from build123d import *

# Parameters (mm, degrees)
SKETCH1_W           = 880
SKETCH1_H           = 580
BOSS_EXTRUDE1_DEPTH = 35
SKETCH2_R           = 50
CUT_EXTRUDE1_DEPTH  = 10
SKETCH3_R           = 30
CUT_EXTRUDE2_DEPTH  = 20
SKETCH4_R           = 15
CUT_EXTRUDE3_DEPTH  = 522
CHAMFER1_SIZE       = 2
SKETCH5_R           = 20
CUT_EXTRUDE4_DEPTH  = 450


with BuildPart() as part:
    # Sketch1 → Boss-Extrude1 (new body)
    with BuildSketch(Plane(origin=(0, 0, 0), x_dir=(1, 0, 0), z_dir=(0, 1, 0))):
        Rectangle(SKETCH1_W, SKETCH1_H)
    extrude(amount=BOSS_EXTRUDE1_DEPTH)

    # Sketch2 → Cut-Extrude1 (cut)
    with BuildSketch(Plane(origin=(0, 35, 0), x_dir=(1, 0, 0), z_dir=(0, 1, 0))):
        with Locations(Location((0, 0, 0), (0, 0, 270))):
            Circle(SKETCH2_R)
    extrude(amount=-CUT_EXTRUDE1_DEPTH, mode=Mode.SUBTRACT)

    # Sketch3 → Cut-Extrude2 (cut)
    with BuildSketch(Plane(origin=(0, 25, 0), x_dir=(1, 0, 0), z_dir=(0, 1, 0))):
        with Locations(Location((0, 0, 0), (0, 0, 270))):
            Circle(SKETCH3_R)
    extrude(amount=-CUT_EXTRUDE2_DEPTH, mode=Mode.SUBTRACT)

    # Sketch4 → Cut-Extrude3 (cut)
    with BuildSketch(Plane(origin=(0, 5, 0), x_dir=(1, 0, 0), z_dir=(0, 1, 0))):
        with Locations(Location((0, 0, 0), (0, 0, 270))):
            Circle(SKETCH4_R)
    extrude(amount=-CUT_EXTRUDE3_DEPTH, mode=Mode.SUBTRACT)

    # Chamfer1
    chamfer1_edges = [part.edges().sort_by_distance(p)[0] for p in [
        (0, 5, -30),
    ]]
    chamfer(chamfer1_edges, length=CHAMFER1_SIZE)

    # Sketch5 → Cut-Extrude4 (cut)
    with BuildSketch(Plane(origin=(0, 35, 0), x_dir=(1, 0, 0), z_dir=(0, 1, 0))):
        with Locations(Location((-340, 200, 0), (0, 0, 270))):
            Circle(SKETCH5_R)
        with Locations(Location((340, 200, 0), (0, 0, 270))):
            Circle(SKETCH5_R)
        with Locations(Location((340, -200, 0), (0, 0, 270))):
            Circle(SKETCH5_R)
        with Locations(Location((-340, -200, 0), (0, 0, 270))):
            Circle(SKETCH5_R)
    extrude(amount=-CUT_EXTRUDE4_DEPTH, mode=Mode.SUBTRACT)


solid = part.part
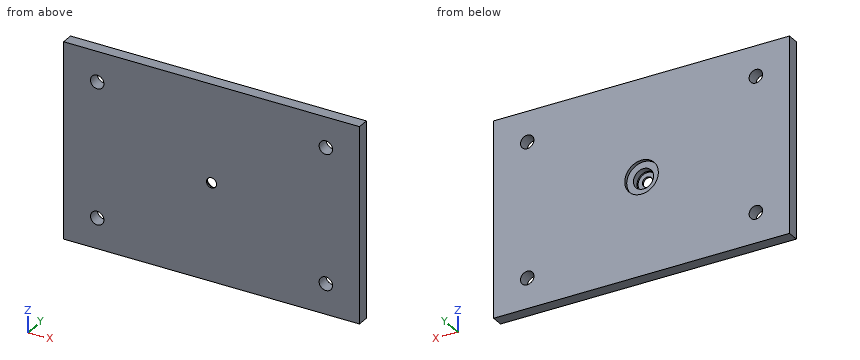
Geometry check sheet. Reference: the model listing, model coordinates, mm. Round coordinates to 2 decimals unless told otherwise and drop trailing zeros. Loops run counter-clockwise (first coordinate to the right, second up) from the corner with the lowest first, then second, coordinate; pieces in that order, holes last.
Item 1: Cross-section at C-C on x = 340. Record the boundary of the cut face in (y, z).
Item 2: Cross-section at A-A on z = 0. Record the boundary of the cut face in (x, y).
Item 3: Thickness scan on line 1 (X direction, y = 16, z = -200); line 2 (X direction, y = 32, z = 0); line 3 (Z direction, x = 335.5, y = 32). Record the ranges inside material, lowest first.
Item 4: Cross-section at D-D on x = 0. Record the boundary of the cut face in (y, z), then the cut area to 3 significant figures.
Item 5: Cross-section at B-B on z = 200. Record the boundary of the cut face in (x, y), then the cut area to 3 significant figures.
Item 6: Gauge pin test, flat end, axial feed: pin 1 (17 mm diameter, centred on x = 3, z = -3.5, fed in from +Y). Record the tip position at first contact, or that the pin passes through.
Answer sheet:
1. outline: (0, -290) - (35, -290) - (35, -220) - (0, -220) - close; (0, -180) - (35, -180) - (35, 180) - (0, 180) - close; (0, 220) - (35, 220) - (35, 290) - (0, 290) - close
2. outline: (-440, 0) - (-15, 0) - (-15, 5) - (-28, 5) - (-30, 7) - (-30, 25) - (-50, 25) - (-50, 35) - (-440, 35) - close; (15, 0) - (440, 0) - (440, 35) - (50, 35) - (50, 25) - (30, 25) - (30, 7) - (28, 5) - (15, 5) - close
3. line 1: x = -440 to -360, -320 to 320, 360 to 440
3. line 2: x = -440 to -50, 50 to 440
3. line 3: z = -290 to -219.49, -180.51 to 180.51, 219.49 to 290
4. outline: (0, -290) - (35, -290) - (35, -50) - (25, -50) - (25, -30) - (7, -30) - (5, -28) - (5, -15) - (0, -15) - close; (0, 15) - (5, 15) - (5, 28) - (7, 30) - (25, 30) - (25, 50) - (35, 50) - (35, 290) - (0, 290) - close
4. area: 18,000 mm2
5. outline: (-440, 0) - (-360, 0) - (-360, 35) - (-440, 35) - close; (-320, 0) - (320, 0) - (320, 35) - (-320, 35) - close; (360, 0) - (440, 0) - (440, 35) - (360, 35) - close
5. area: 28,000 mm2
6. pin 1: passes through
